Here's how the part is built. I have some questions about the finished solid (model axes, mm). A direction names the side the tool comes from. Give positions to 0.01 mm unless a question says otherwise; leave off trailing zeros. Loops run counter-clockwise (first coordinate to the right, second up) from the corner with the lowest first, then second, coordinate; pieces in that order, holes last. Notation, with made-up numbers: (-12, 86.5) - (33, 86.5) arc R13 cw to (33, 103.5) - close; hole circle Ø1 at (-4.5, -28). An arc over 180 degrees is marked (long way). Return JSON: item names as keys, results as strings. Group by question number.
(1) If we section it at B-B (y = 0): Please give me the cut outline in (x, z).
(2) For P1, Ø12, axis at x = 23, z = -43, coming from the -Y side; P2, Ø2, axis at x = 12.5, z = -0.5, coming from the -Y side; P3, Ø20, axis at y = 7, z = -25, coming from the -X side, each with a flat end and sliding along its axis, tell me the tip position at first contact or that it passes through.
(3) I need wall thicknesses on probe 1 along Y at (x, z) = (15, 11.5); probe 2 along Z at (x, y) = (23.5, 0); probe 3 along X at (y, z) = (4, -19.5). Which ranges of each line are inside material? Lowest first, please. Write a range as [from, to].
(4) If we section it at C-C (x = 21): Please give me the cut outline in (y, z), then the cut area to 3 significant figures.
(5) If we section it at A-A (z = -35): Please give me the cut outline in (x, y), then the cut area to 3 significant figures.
(6) If we mould it in two halves opening along Y, with no side actions, what happens to faces 1 (the flat face through (3, 50, 10)), 2 (the flat face through (2, -50, 10)), 3 (the cylindrical face through (13.16, -28.31, 7.6)), 4 (the flat face through (15, 0, -27))? For each: released by +Y, released by -Y, zero draft, split by the parting line, or undercut.
(7) If we section it at D-D (y = -30): Please give me the cut outline in (x, z), then the cut area to 4 significant figures.
(8) On a 3-axis mill with a long thin cutter (end or side, diameter ignored), from which of +Z, -Z, +X, -X, +Y, -Y can I reach the whole of each face in a straight line? I mean faces 5 (the flat face through (23, 20, -25)), 6 (the cylindrical face through (22.4, 1.63, -42.32)), 7 (the flat face through (23, -20, -25)). Say none if no direction works.
```python
from build123d import *

# Parameters (mm, degrees)
F1_DEPTH = 15
F2_W     = 40
F2_H     = 50
F3_DEPTH = 15
F4_R     = 5
F5_SIZE  = 5
F6_R     = 7.5
F7_DEPTH = 25
F8_R     = 2.5
F9_DEPTH = 25


with BuildPart() as f1:
    # F0 (on Top) → F1 (new body)
    with BuildSketch(Plane.XY):
        with BuildLine():
            Line((30, 50), (-25, 50))
            ThreePointArc((-25, 50), (-28.5355339059, 48.5355339059), (-30, 45))
            Line((-30, 45), (-30, -45))
            ThreePointArc((-30, -45), (-28.5355339059, -48.5355339059), (-25, -50))
            Line((-25, -50), (30, -50))
            Line((30, -50), (30, 50))
        make_face()
    extrude(amount=F1_DEPTH)

    # F2 (on face) → F3 (join)
    with BuildSketch(Plane.YZ.offset(30)):
        with Locations((0, -25)):
            Rectangle(F2_W, F2_H)
    extrude(amount=-F3_DEPTH)

    # F4
    f4_edges = [f1.edges().sort_by_distance(p)[0] for p in [
        (22.5, 20, 0),
        (15, 0, 0),
        (22.5, 20, -50),
        (22.5, -20, -50),
        (22.5, -20, 0),
    ]]
    fillet(f4_edges, radius=F4_R)

    # F5
    f5_edges = [f1.edges().sort_by_distance(p)[0] for p in [
        (2.5, 50, 0),
    ]]
    chamfer(f5_edges, length=F5_SIZE)

    # F6 (on face) → F7 (cut)
    with BuildSketch(Plane(origin=(15, 0, 0), x_dir=(0, -1, 0), z_dir=(-1, 0, 0))):
        with Locations((0, -35)):
            Circle(F6_R)
    extrude(amount=-F7_DEPTH, mode=Mode.SUBTRACT)

    # F8 (on face) → F9 (cut)
    with BuildSketch(Plane.XY.offset(15)):
        with Locations((-15, -30)):
            Circle(F8_R)
        with Locations((15, -30)):
            Circle(F8_R)
        with Locations((15, 30)):
            Circle(F8_R)
        with Locations((-15, 30)):
            Circle(F8_R)
    extrude(amount=-F9_DEPTH, mode=Mode.SUBTRACT)


solid = f1.part
```
Values:
{
 "1": {"outline": "(-30, 5) - (-25, 0) - (10, 0) arc R5 cw to (15, -5) - (15, -27.5) - (30, -27.5) - (30, 15) - (-30, 15) - close; (15, -50) - (30, -50) - (30, -42.5) - (15, -42.5) - close"},
 "2": {"P1": "y = -20", "P2": "y = -45.5", "P3": "x = 15"},
 "3": {"probe 1": "[-50, -32.5], [-27.5, 27.5], [32.5, 50]", "probe 2": "[-50, -42.5], [-27.5, 15]", "probe 3": "[15, 30]"},
 "4": {"outline": "(-50, 5) - (-45, 0) - (-25, 0) arc R5 cw to (-20, -5) - (-20, -45) arc R5 ccw to (-15, -50) - (15, -50) arc R5 ccw to (20, -45) - (20, -5) arc R5 cw to (25, 0) - (45, 0) - (50, 5) - (50, 15) - (-50, 15) - close; hole circle Ø15 at (0, -35)", "area": "3,300 mm2"},
 "5": {"outline": "(15, -20) - (30, -20) - (30, -7.5) - (15, -7.5) - close; (15, 7.5) - (30, 7.5) - (30, 20) - (15, 20) - close", "area": "375 mm2"},
 "6": {"face 1": "released by +Y", "face 2": "released by -Y", "face 3": "undercut", "face 4": "zero draft"},
 "7": {"outline": "(-30, 5) - (-25, 0) - (-17.5, 0) - (-17.5, 15) - (-30, 15) - close; (-12.5, 0) - (12.5, 0) - (12.5, 15) - (-12.5, 15) - close; (17.5, 0) - (30, 0) - (30, 15) - (17.5, 15) - close", "area": "737.5 mm2"},
 "8": {"face 5": "-Z, +X, -X, +Y", "face 6": "+X, -X", "face 7": "-Z, +X, -X, -Y"}
}
